from build123d import *

# Parameters (mm, degrees)
SKETCH1_W           = 140
SKETCH1_H           = 20
BOSS_EXTRUDE1_DEPTH = 10
SKETCH2_W           = 80
SKETCH2_H           = 20
CUT_EXTRUDE1_DEPTH  = 1
SKETCH3_R           = 2.75
CUT_EXTRUDE2_DEPTH  = 9
SKETCH4_R           = 5
CUT_EXTRUDE3_DEPTH  = 6
SKETCH5_R           = 1.65
CUT_EXTRUDE4_DEPTH  = 10


with BuildPart() as part:
    # Sketch1 → Boss-Extrude1 (new body)
    with BuildSketch(Plane(origin=(0, 0, 0), x_dir=(1, 0, 0), z_dir=(0, 1, 0))):
        Rectangle(SKETCH1_W, SKETCH1_H)
    extrude(amount=BOSS_EXTRUDE1_DEPTH)

    # Sketch2 → Cut-Extrude1 (cut)
    with BuildSketch(Plane(origin=(0, 10, 0), x_dir=(1, 0, 0), z_dir=(0, 1, 0))):
        Rectangle(SKETCH2_W, SKETCH2_H)
    extrude(amount=-CUT_EXTRUDE1_DEPTH, mode=Mode.SUBTRACT)

    # Sketch3 → Cut-Extrude2 (cut)
    with BuildSketch(Plane(origin=(0, 9, 0), x_dir=(1, 0, 0), z_dir=(0, 1, 0))):
        with Locations(Location((31, 0, 0), (0, 0, 270))):
            Circle(SKETCH3_R)
        with Locations(Location((-31, 0, 0), (0, 0, 270))):
            Circle(SKETCH3_R)
    extrude(amount=-CUT_EXTRUDE2_DEPTH, mode=Mode.SUBTRACT)

    # Sketch4 → Cut-Extrude3 (cut)
    with BuildSketch(Plane(origin=(0, 9, 0), x_dir=(1, 0, 0), z_dir=(0, 1, 0))):
        with Locations(Location((31, 0, 0), (0, 0, 270))):
            Circle(SKETCH4_R)
        with Locations(Location((-31, 0, 0), (0, 0, 270))):
            Circle(SKETCH4_R)
    extrude(amount=-CUT_EXTRUDE3_DEPTH, mode=Mode.SUBTRACT)

    # Sketch5 → Cut-Extrude4 (cut)
    with BuildSketch(Plane(origin=(0, 10, 0), x_dir=(1, 0, 0), z_dir=(0, 1, 0))):
        with Locations(Location((-50, -3, 0), (0, 0, 270))):
            Circle(SKETCH5_R)
        with Locations(Location((50, -3, 0), (0, 0, 270))):
            Circle(SKETCH5_R)
    extrude(amount=-CUT_EXTRUDE4_DEPTH, mode=Mode.SUBTRACT)


solid = part.part
Input: part model. Units: mm. Frame: model coordinates. A direction names the side the tool comes from. Round coordinates to 2 decimals unless told otherwise and drop trailing zeros. Order: outer loops, then holes, each group sorted by start corner. A loop starts at its lowest first (then second) coordinate and runs counter-clockwise, first axis right, second up. Notation, with made-up numbers: (79.5, 72) - (111.5, 72) arc R36 ccw to (111.5, 106) - close; hole circle Ø6 at (-14, 46.5). An arc over 180 degrees is marked (long way). Use a Markdown table: item, result.
1. Material intervals for probe 1 along X at (y, z) = (6.7, 0); probe 2 along X at (y, z) = (0.8, 0); probe 3 along X at (y, z) = (5, 3), sorted ascending.
Evaluation:
| item | result |
|---|---|
| probe 1 | -70 to -36, -26 to 26, 36 to 70 |
| probe 2 | -70 to -33.75, -28.25 to 28.25, 33.75 to 70 |
| probe 3 | -70 to -51.65, -48.35 to -35, -27 to 27, 35 to 48.35, 51.65 to 70 |
2. Mould query, pull axis X, two halves, no side actions, for faces 1 (the face through (70, 5, 0)), 2 (the face through (-48.61, 5.07, 3.89)), 3 (the face through (-1, 9, 0)), 4 (the face through (-70, 5, 0)). Classes: +X half, -X half, draft (parallel to the pull), parting line (faces both ways), or undercut.
Evaluation:
| item | result |
|---|---|
| face 1 | +X half |
| face 2 | undercut |
| face 3 | undercut |
| face 4 | -X half |
3. Section A-A on z = 0. Return the cut outline in (x, y), then the cut area to 3 significant figures.
Evaluation:
| item | result |
|---|---|
| outline | (-70, 0) - (-33.75, 0) - (-33.75, 3) - (-36, 3) - (-36, 9) - (-40, 9) - (-40, 10) - (-70, 10) - close; (-28.25, 0) - (28.25, 0) - (28.25, 3) - (26, 3) - (26, 9) - (-26, 9) - (-26, 3) - (-28.25, 3) - close; (33.75, 0) - (70, 0) - (70, 10) - (40, 10) - (40, 9) - (36, 9) - (36, 3) - (33.75, 3) - close |
| area | 1,170 mm^2 |
4. First-contact query: pin 1 (6 mm diameter, centred on x = -30, z = -2.5, fed in from +Y); pin 2 (2 mm diameter, centred on x = 50, z = 3, fed in from +Y). Flat tips, straight axial feed; report the tip coordinate or a pass-through.
Evaluation:
| item | result |
|---|---|
| pin 1 | y = 9 |
| pin 2 | through |
5. Section D-D on x = -31. Return the cut outline in (y, z), then the cut area to 4 significant figures.
Evaluation:
| item | result |
|---|---|
| outline | (0, -10) - (9, -10) - (9, -5) - (3, -5) - (3, -2.75) - (0, -2.75) - close; (0, 2.75) - (3, 2.75) - (3, 5) - (9, 5) - (9, 10) - (0, 10) - close |
| area | 103.5 mm^2 |
6. Section B-B on x = 50. Return the cut outline in (y, z), then the cut area to 3 significant figures.
Evaluation:
| item | result |
|---|---|
| outline | (0, -10) - (10, -10) - (10, 1.35) - (0, 1.35) - close; (0, 4.65) - (10, 4.65) - (10, 10) - (0, 10) - close |
| area | 167 mm^2 |
7. Access query for faces 5 (the face through (28.8, 3, 2.2)), 6 (the face through (-1, 5, 10)). Directions: +Z, -Z, +X, -X, +Y, -Y. A direction counts if a zero-diameter tool reaches every point of the face in a straight line with its end or side. Return the directions, or none.
Evaluation:
| item | result |
|---|---|
| face 5 | +Y |
| face 6 | +Z, +X, -X, +Y, -Y |
8. Section C-C on y = 1.5. Return the cut outline in (x, z).
Evaluation:
| item | result |
|---|---|
| outline | (-70, -10) - (70, -10) - (70, 10) - (-70, 10) - close; hole circle Ø3.3 at (-50, 3); hole circle Ø5.5 at (-31, 0); hole circle Ø5.5 at (31, 0); hole circle Ø3.3 at (50, 3) |
